Input: part model. Units: mm. Frame: model coordinates. A direction names the side the tool comes from. Give positions to 0.01 mm unless a question says otherwise; leave off trailing zeros. Write each loop counter-clockwise with the first axis right and the second up, starting at its lowest first coordinate (ties: lowest second). Pieces come first, ordered by that corner, then holes. Notation, with made-up numbers: (-27, 8.25) -> (-2, 8.25) arc R11 ccw to (-2, 17.25) -> close; hole circle Ø8 at (-22, 44.5). An arc over 180 degrees is marked (long way). Return JSON: item names as keys, results as strings. Group by question number.
Item 1: Section B-B, the plane x = -26.5. Return loops of the section in (y, z).
Item 2: Pin query (flat end, axial travel): P1, Ø6, axis at x = 486.5, y = -2.5, coming from the +Z side; P2, Ø1, axis at y = -190.5, z = 58, coming from the -X side; P3, Ø6, axis at x = 491, y = -12.5, coming from the +Z side. Return the tip coordinate at first contact, or that it passes through.
Item 3: Section A-A, the plane x = 1288.5. Return loops of the section in (y, z), then the cut area to 3 significant figures.
Item 4: Line query: line 1 (Y direction, x = 1270, z = -85); line 2 (Y direction, x = 736, z = -104); line 3 (Z direction, x = 744, y = -177.5). Output: solid intervals per line, ascending. Write a range as [from, to].
Item 5: Set-up query: faces 1 (the face through (-151, -102.108, 1)), 2 (the face through (-151, -1, 102.108)), 3 (the face through (-151, -1, -102.108)), 4 (the face through (-151, 102.108, 1)). Return all of +Z, -Z, +X, -X, +Y, -Y with unobstructed straight access to the full face (end or side cutting, diameter ignored); none if empty.
from build123d import *

# Parameters (mm, degrees)
LOFT1_START         = -125.7300001
LOFT1_DEPTH         = 251.4600001
LOFT1_START_2       = -371
LOFT1_2_DEPTH       = 475
SKETCH6_W           = 204.216
SKETCH6_H           = 204.216
BOSS_EXTRUDE1_DEPTH = 306.324
SKETCH8_W           = 251.46
SKETCH8_H           = 251.46
BOSS_EXTRUDE2_DEPTH = 377.19


with BuildPart() as part:
    # Loft1: read off the stored shape, not the designer's step
    # Loft1 outline → Loft1 (new body)
    with BuildSketch(Plane.XY.offset(LOFT1_START)):
        with BuildLine():
            Line((1021.373155762, -369.703305112), (1021.373155762, -118.243305112))
            add(Edge.make_bspline(
                [(0, 102.108), (196.914895518, 111.82689324), (392.936444227, 69.537154328), (708.143629326, -92.279435597), (864.402326567, -125.990726792), (1021.373155762, -118.243305112)],
                knots=[0, 0, 0, 0, 0.556436391, 0.556436391, 1, 1, 1, 1], degree=3))
            Line((0, 102.108), (0, -102.108))
            add(Edge.make_bspline(
                [(0, -102.108), (196.914895518, -101.151867047), (392.936444227, -152.204366245), (708.143629326, -329.768956171), (864.402326567, -370.465487079), (1021.373155762, -369.703305112)],
                knots=[0, 0, 0, 0, 0.556436391, 0.556436391, 1, 1, 1, 1], degree=3))
        make_face()
    extrude(amount=LOFT1_DEPTH)

    # Loft1 2 outline → Loft1 2 (cut)
    with BuildSketch(Plane(origin=(0, 0, 0), x_dir=(1, 0, 0), z_dir=(0, 1, 0)).offset(LOFT1_START_2)):
        with BuildLine():
            Line((0, 125.7300001), (0, 102.108))
            add(Edge.make_bspline(
                [(0, 102.108), (196.914895518, 106.489380143), (392.936444227, 110.870760287), (708.143629326, 118.744760287), (864.402326567, 122.237380143), (1021.373155762, 125.73)],
                knots=[0, 0, 0, 0, 0.556436391, 0.556436391, 1, 1, 1, 1], degree=3))
            Line((1021.373155762, 125.73), (0, 125.7300001))
        make_face()
        with BuildLine():
            add(Edge.make_bspline(
                [(0, -102.108), (196.914895518, -106.489380143), (392.936444227, -110.870760287), (708.143629326, -118.744760287), (864.402326567, -122.237380143), (1021.373155762, -125.73)],
                knots=[0, 0, 0, 0, 0.556436391, 0.556436391, 1, 1, 1, 1], degree=3))
            Line((0, -102.108), (0, -125.73))
            Line((0, -125.73), (1021.373155762, -125.73))
        make_face()
    extrude(amount=LOFT1_2_DEPTH, mode=Mode.SUBTRACT)

    # Sketch6 → Boss-Extrude1 (add)
    with BuildSketch(Plane(origin=(0, 0, 0), x_dir=(0, 0, -1), z_dir=(1, 0, 0))):
        Rectangle(SKETCH6_W, SKETCH6_H)
    extrude(amount=-BOSS_EXTRUDE1_DEPTH)

    # Sketch8 → Boss-Extrude2 (add)
    with BuildSketch(Plane(origin=(1021.373155762, 0, 0), x_dir=(0, 0, -1), z_dir=(1, 0, 0))):
        with Locations((0, -243.973305112)):
            Rectangle(SKETCH8_W, SKETCH8_H)
    extrude(amount=BOSS_EXTRUDE2_DEPTH)


solid = part.part
Answer below:
{
 "1": {"outline": "(-102.11, -102.11) -> (102.11, -102.11) -> (102.11, 102.11) -> (-102.11, 102.11) -> close"},
 "2": {"P1": "stops at z = 113.31", "P2": "stops at x = 443.16", "P3": "stops at z = 113.42"},
 "3": {"outline": "(-369.7, -125.73) -> (-118.24, -125.73) -> (-118.24, 125.73) -> (-369.7, 125.73) -> close", "area": "63,200 mm2"},
 "4": {"line 1": "y = [-369.7, -118.24]", "line 2": "y = [-324.78, -86.22]", "line 3": "z = [-119.47, 119.47]"},
 "5": {"face 1": "+Z, -Z, -X, -Y", "face 2": "+Z, -X, +Y, -Y", "face 3": "-Z, -X, +Y, -Y", "face 4": "+Z, -Z, -X, +Y"}
}
